Input: part model. Units: mm. Frame: model coordinates. Face numbers are marked on the shaded views. A direction names the side the tool comes from. Give positions to 0.01 mm unless a question says otherwise; leave off trailing zeros. Write each loop counter-clockwise with the first axis right and the second up, starting at its lowest first coordinate (ties: lowest second). Pieces come first, ordered by that corner, then holes. Notation, with made-up numbers: (57, 80.5) - (71, 80.5) arc R29 cw to (71, 117.5) - close; hole circle Ø3 at (5.5, 51). An arc over 180 degrees is marked (long way). Answer as CSV lines item,"result".
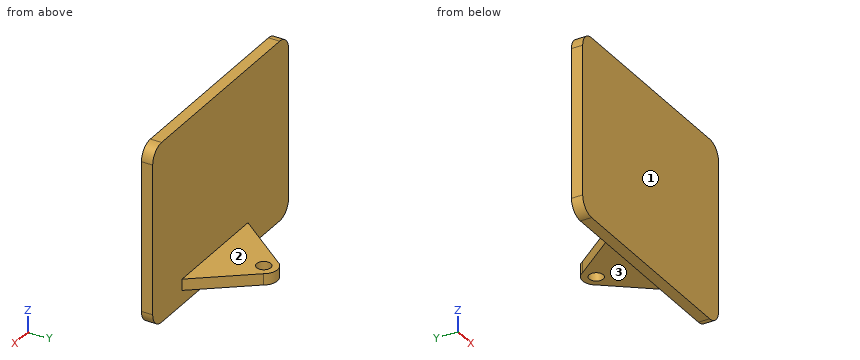
Autodesk Inventor part; units mm, degrees
ref_plane "YZ Plane" through (0, 0, 0) normal (1, 0, 0) x (0, 1, 0)
ref_plane "XZ Plane" through (0, 0, 0) normal (0, 1, 0) x (-1, 0, 0)
ref_plane "XY Plane" through (0, 0, 0) normal (0, 0, 1) x (1, 0, 0)
ref_plane "Work Plane1" through (0, 0, 0) normal (0, 0, 1) x (1, 0, 0)
sketch "Sketch1" plane through (0, 0, 0) normal (0, 0, 1) x (1, 0, 0)
  circle A0 centre (0, -6.2841) radius 1.4986
  arc A1 (-2.5077, -7.7319) -> (2.5077, -7.7319) centre (0, -6.2841) ccw
  line L0 (-2.5077, -7.7319) -> (-11.746, 4.0347)
  line L1 (11.746, 4.0347) -> (-11.746, 4.0347)
  line L2 (11.746, 4.0347) -> (2.5077, -7.7319)
  circle A2 centre (0, -6.2841) radius 1.4986
  line L3 (-11.746, 4.0347) -> (-3.6444, -6.2841)
  line L4 (3.6444, -6.2841) -> (11.746, 4.0347)
  line L5 (11.746, 4.0347) -> (-11.746, 4.0347)
  line L6 (2.5077, -4.8363) -> (11.7464, -16.6034)
  line L7 (-2.5077, -4.8363) -> (-11.7464, -16.6034)
  line L8 (-11.7464, -16.6034) -> (11.7464, -16.6034)
  arc A3 (2.5077, -4.8363) -> (-2.5077, -4.8363) centre (0, -6.2841) ccw
  point P0 (0, 0)
  dimension "d0" = 14.9606
  dimension "d1" = 14.9606
extrude "Extrusion1" add sketch "Sketch1" along normal blind 2.3813 contours L0 L7 A3 L6 L2 A1 | A1 L2 L6 L8 L7 L0
sketch "Sketch2" plane through (-11.7464, -16.6034, 0) normal (0, -1, 0) x (1, 0, 0)
  line L0 (5.9964, 35) -> (26.2464, 35)
  line L1 (20.4964, -2.75) -> (29.2464, -2.75)
  line L2 (-7.5036, -3) -> (1.4964, -3)
  line L3 (-14.5036, 16.05) -> (-14.5036, 26.8)
  line L4 (33.9964, 15.95) -> (33.9964, 5)
  line L5 (-14.5036, 26.8) -> (-14.5036, -3)
  line L6 (-14.5036, -3) -> (33.9964, -3)
  line L7 (33.9964, -3) -> (33.9964, 35)
  line L8 (33.9964, 35) -> (-14.5036, 35)
  line L9 (-14.5036, -3) -> (-14.5036, 35)
  point P0 (11.7464, 0)
extrude "Extrusion2" add sketch "Sketch2" along normal blind 2.3813
fillet "Fillet1" radius 3.175 1 edges at (-26.25, -17.794, -3)
fillet "Fillet2" radius 3.175 1 edges at (-26.25, -17.794, 35)
fillet "Fillet3" radius 3.175 1 edges at (22.25, -17.794, 35)
fillet "Fillet4" radius 3.175 1 edges at (22.25, -17.794, -3)
properties part number "headtilt-base"
Item 1: Contact query for flat-ended pins moving along their axis: pin 1 (6.5 mm diameter, centred on x = -1, y = -11, fed in from -Z); pin 2 (19 mm diameter, centred on x = -11.5, z = 18, fed in from +Y). Output: stop coordinate, or through.
The answers:
pin 1,"z = 0"
pin 2,"y = -16.6"
Item 2: Ray query, line 1 (Y direction, x = 0, z = 1.35); line 2 (Z direction, x = 1, y = -14.75); line 3 (Y direction, x = -9, z = 7). Return the intervals inside material, ascending. Write a range as from..to.
The answers:
line 1,"-18.98..-7.78, -4.79..-3.39"
line 2,"0..2.38"
line 3,"-18.98..-16.6"
Item 3: Reachability of the marked faces 1, 2 and 3 from +Z, -Z, +X, -X, +Y, -Y: full face, straight path, thin tool, end or side. Return the list, or none.
The answers:
face 1,"+Z, -Z, +X, -X, -Y"
face 2,"+Z, +X, -X, +Y"
face 3,"-Z, +X, -X, +Y"
Item 4: Cut plane A-A on y = -7.25. Return the cut outline in (x, z).
The answers:
outline,"(-4.4, 0) - (-1.15, 0) - (-1.15, 2.38) - (-4.4, 2.38) - close; (1.15, 0) - (4.4, 0) - (4.4, 2.38) - (1.15, 2.38) - close"
Item 5: Cut plane B-B on x = 0. Return the cut outline in (y, z).
The answers:
outline,"(-18.98, -3) - (-16.6, -3) - (-16.6, 0) - (-7.78, 0) - (-7.78, 2.38) - (-16.6, 2.38) - (-16.6, 35) - (-18.98, 35) - close; (-4.79, 0) - (-3.39, 0) - (-3.39, 2.38) - (-4.79, 2.38) - close"
Item 6: Cut plane C-C on z = 4. Return the cut outline in (x, y).
The answers:
outline,"(-26.25, -18.98) - (22.25, -18.98) - (22.25, -16.6) - (-26.25, -16.6) - close"
Item 7: Cut plane D-D on y = -14.25. Return the cut outline in (x, z), plus the area to 3 significant figures.
The answers:
outline,"(-9.9, 0) - (9.9, 0) - (9.9, 2.38) - (-9.9, 2.38) - close"
area,"47.1 mm²"
